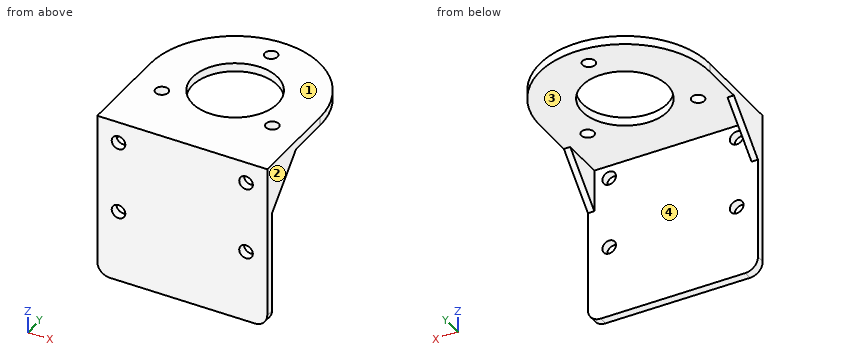
from build123d import *

# Parameters (mm, degrees)
SKETCH1_R           = 1.5
SKETCH1_R_2         = 10
BOSS_EXTRUDE1_DEPTH = 2
SKETCH2_W           = 40
SKETCH2_H           = 2
BOSS_EXTRUDE2_DEPTH = 37
FILLET1_R           = 3
SKETCH3_R           = 1.6
CUT_EXTRUDE1_DEPTH  = 59.043087444
RIB2_DEPTH          = 1.5


# Read off the part's stored shape, not the designer's step: Rib2
with BuildPart() as part:
    # Sketch1 → Boss-Extrude1 (new body)
    with BuildSketch(Plane.XY):
        with BuildLine():
            Line((-20, 0), (-20, -22))
            Line((-20, -22), (20, -22))
            Line((20, -22), (20, 0))
            ThreePointArc((20, 0), (0, 20), (-20, 0))
        make_face()
        with Locations((0, 15)):
            Circle(SKETCH1_R, mode=Mode.SUBTRACT)
        with Locations((12.990381057, -7.5)):
            Circle(SKETCH1_R, mode=Mode.SUBTRACT)
        with Locations((-12.990381057, -7.5)):
            Circle(SKETCH1_R, mode=Mode.SUBTRACT)
        Circle(SKETCH1_R_2, mode=Mode.SUBTRACT)
    extrude(amount=BOSS_EXTRUDE1_DEPTH)

    # Sketch2 → Boss-Extrude2 (add)
    with BuildSketch(Plane(origin=(0, 0, 0), x_dir=(-1, 0, 0), z_dir=(0, 0, -1))):
        with Locations((0, -21)):
            Rectangle(SKETCH2_W, SKETCH2_H)
    extrude(amount=BOSS_EXTRUDE2_DEPTH)

    # Fillet1
    fillet1_edges = [part.edges().sort_by_distance(p)[0] for p in [
        (-20, -21, -37),
        (20, -21, -37),
    ]]
    fillet(fillet1_edges, radius=FILLET1_R)

    # Sketch3 → Cut-Extrude1 (cut, through all)
    with BuildSketch(Plane(origin=(0, -20, 0), x_dir=(1, 0, 0), z_dir=(0, 1, 0))):
        with Locations(Location((15, 20, 0), (0, 0, 180))):
            Circle(SKETCH3_R)
        with Locations(Location((15, 3, 0), (0, 0, 180))):
            Circle(SKETCH3_R)
        with Locations((-15, 3)):
            Circle(SKETCH3_R)
        with Locations((-15, 20)):
            Circle(SKETCH3_R)
    extrude(amount=-CUT_EXTRUDE1_DEPTH, mode=Mode.SUBTRACT)

    # Rib2 outline → Rib2 (add)
    with BuildSketch(Plane(origin=(-20, 0, 0), x_dir=(0, 0, -1), z_dir=(1, 0, 0))):
        Polygon((10, -20), (0, -10), (0, -20), align=None)
    rib2 = extrude(amount=RIB2_DEPTH)

    # Mirror1: Rib2 across plane
    add(rib2.mirror(Plane(origin=(0, 0, 0), x_dir=(0, 0, 1), z_dir=(1, 0, 0))))


solid = part.part
Model file for the job. Use its own axes, mm. Face numbers are marked on the shaded views. Round coordinates to 2 decimals unless told otherwise and drop trailing zeros. Order: outer loops, then holes, each group sorted by start corner. A loop starts at its lowest first (then second) coordinate and runs counter-clockwise, first axis right, second up.
(1) Pull direction X, two halves, no side cores. Call the marked faces 1, 2, 3 and 4: released by +X, released by -X, zero draft, split by the parting line, or undercut.
(2) Band-saw the part on D-D (y = -7.5). List the corners of the cut face in (x, z), then the cut area to 3 significant figures.
(3) Drill centre lines: line 1 (Z direction, x = -15, y = -21); line 2 (Y direction, x = 0, z = 0.7); line 3 (Z direction, x = 9, y = -5.5). Where is each one in solid material? Low to high.
(4) Band-saw the part on A-A (z = -3). List the corners of the cut face in (x, y), then the cut area to 3 significant figures.
(5) Band-saw the part on C-C (y = -16.5). List the corners of the cut face in (x, z), then the cut area to 3 significant figures.
(6) Band-saw the part on B-B (y = 6). List the corners of the cut face in (x, z), then the cut area to 3 significant figures.
(7) Pin check, flat tips, straight feed: pin 1 (4 mm diameter, centred on x = 12.99, y = -7.5, fed in from -Z); pin 2 (18.5 mm diameter, centred on x = -2.5, z = -25.5, fed in from +Y). Stop position of each tip, or through.
Verdict:
1. face 1: zero draft
1. face 2: released by +X
1. face 3: undercut
1. face 4: undercut
2. outline: (-20, 0) - (-14.49, 0) - (-14.49, 2) - (-20, 2) - close; (-11.49, 0) - (-6.61, 0) - (-6.61, 2) - (-11.49, 2) - close; (6.61, 0) - (11.49, 0) - (11.49, 2) - (6.61, 2) - close; (14.49, 0) - (20, 0) - (20, 2) - (14.49, 2) - close
2. area: 41.5 mm2
3. line 1: z = -37 to -21.6, -18.4 to -4.6, -1.4 to 2
3. line 2: y = -22 to -10, 10 to 13.5, 16.5 to 20
3. line 3: z = 0 to 2
4. outline: (-20, -22) - (-16.6, -22) - (-16.6, -20) - (-18.5, -20) - (-18.5, -13) - (-20, -13) - close; (-13.4, -22) - (13.4, -22) - (13.4, -20) - (-13.4, -20) - close; (16.6, -22) - (20, -22) - (20, -13) - (18.5, -13) - (18.5, -20) - (16.6, -20) - close
4. area: 88.2 mm2
5. outline: (-20, -6.5) - (-18.5, -6.5) - (-18.5, 0) - (18.5, 0) - (18.5, -6.5) - (20, -6.5) - (20, 2) - (-20, 2) - close
5. area: 99.5 mm2
6. outline: (-19.08, 0) - (-8, 0) - (-8, 2) - (-19.08, 2) - close; (8, 0) - (19.08, 0) - (19.08, 2) - (8, 2) - close
6. area: 44.3 mm2
7. pin 1: stops at z = 0
7. pin 2: stops at y = -20
